```python
from build123d import *

# Parameters (mm, degrees)
SKETCH_1_W          = 10.622879294
SKETCH_1_H          = 7.171059062
EXTRUDE_1_DEPTH     = 6
EXTRUDE_2_DEPTH     = 6
SKETCH_3_W          = 1.75
SKETCH_3_H          = 1.75
CUT_EXTRUDE_1_DEPTH = 4


with BuildPart() as part:
    # 草图1 → 凸台-拉伸1 (new body)
    with BuildSketch(Plane.XY):
        with Locations((2.891532243, 0.829398912)):
            Rectangle(SKETCH_1_W, SKETCH_1_H)
    extrude(amount=EXTRUDE_1_DEPTH)

    # 草图2 → 凸台-拉伸2 (add)
    with BuildSketch(Plane.XY.offset(6)):
        with BuildLine():
            Line((1.830465057, 2.928210333), (3.810000549, 2.928210333))
            ThreePointArc((3.810000549, 2.928210333), (4.51710733, 2.635317114), (4.810000549, 1.928210333))
            Line((4.810000549, 1.928210333), (4.810000549, -0.252824237))
            ThreePointArc((4.810000549, -0.252824237), (4.51710733, -0.959931018), (3.810000549, -1.252824237))
            Line((3.810000549, -1.252824237), (1.830465057, -1.252824237))
            ThreePointArc((1.830465057, -1.252824237), (1.123358276, -0.959931018), (0.830465057, -0.252824237))
            Line((0.830465057, -0.252824237), (0.830465057, 1.928210333))
            ThreePointArc((0.830465057, 1.928210333), (1.123358276, 2.635317114), (1.830465057, 2.928210333))
        make_face()
    extrude(amount=EXTRUDE_2_DEPTH)

    # 草图3 → 切除-拉伸1 (cut)
    with BuildSketch(Plane(origin=(0, 0, 0), x_dir=(-1, 0, 0), z_dir=(0, 0, -1))):
        with Locations((-2.744430707, 0.686146252)):
            Rectangle(SKETCH_3_W, SKETCH_3_H)
    extrude(amount=-CUT_EXTRUDE_1_DEPTH, mode=Mode.SUBTRACT)


solid = part.part
```
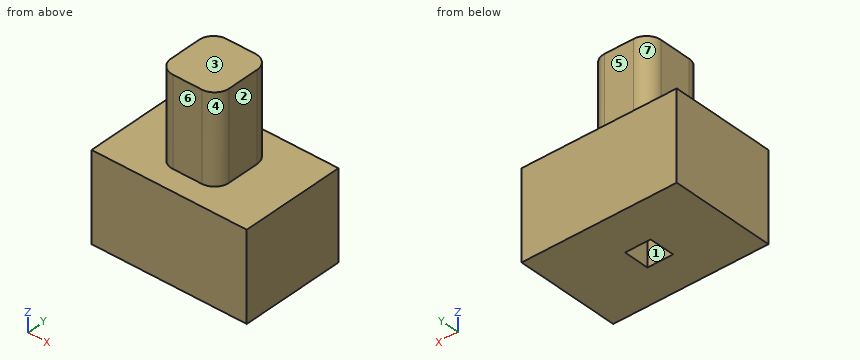
Input: part model. Units: mm. Frame: model coordinates. Face numbers are marked on the shaded views. A direction names the side the tool comes from. Coordinates: 2 decimals unless noted, no trailing zeros. Loops run counter-clockwise (first coordinate to the right, second up) from the corner with the lowest first, then second, coordinate; pieces in that order, holes last. Notation, with made-up numbers: M 3,4.25 L 31,4.25 A26 ccw 31,42.25 Z; hole C 82.5,72 d3. An arc over 180 degrees is marked long. Use a Markdown table: item, result. Add a question column.
1) Line query: L1, parallel to X at y = 0.5, z = 3.5; L2, parallel to Y at x = 3.5, z = 0.5; L3, parallel to X at y = 0.5, z = 9.5. Output: solid intervals per line, ascending. Write a range as from..to.
2) Section A-A, the plane z = 2.5. Return the cut outline in (x, y), plus the area to 3 significant figures.
3) Section C-C, the plane y = 0.25. Return the cut outline in (x, z).
4) Set-up query: the marked faces 4, 5, 6 and 7. Return all of +Z, -Z, +X, -X, +Y, -Y with unobstructed straight access to the full face (end or side cutting, diameter ignored); none if empty.
5) Section D-D, the plane z = 11. Return the cut outline in (x, y), plus the area to 3 significant figures.
6) Draft query along X for the marked faces 1, 2 and 3. Return one class per face: +X half, -X half, draft (parallel to the pull), parting line (faces both ways), or undercut.
7) Pin query (flat end, axial travel): P1, Ø2, axis at x = 3, z = 10, coming from the -Y side; P2, Ø0.9, axis at x = 3, y = 0.5, coming from the -Z side; P3, Ø2.5, axis at y = 1, z = 9, coming from the +X side. Return the tip coordinate at first contact, or that it passes through.
8) Section B-B, the plane x = 3. Return the cut outline in (y, z).
Answer below:
| question | item | result |
|---|---|---|
| 1 | L1 | -2.42..1.87, 3.62..8.2 |
| 1 | L2 | -2.76..-0.19, 1.56..4.41 |
| 1 | L3 | 0.83..4.81 |
| 2 | outline | M -2.42,-2.76 L 8.2,-2.76 L 8.2,4.41 L -2.42,4.41 Z; hole M 1.87,-0.19 L 3.62,-0.19 L 3.62,1.56 L 1.87,1.56 Z |
| 2 | area | 73.1 mm2 |
| 3 | outline | M -2.42,0 L 1.87,0 L 1.87,4 L 3.62,4 L 3.62,0 L 8.2,0 L 8.2,6 L 4.81,6 L 4.81,12 L 0.83,12 L 0.83,6 L -2.42,6 Z |
| 4 | face 4 | +Z, +X, -Y |
| 4 | face 5 | +Z, +X, -X, +Y |
| 4 | face 6 | +Z, +X, -X, -Y |
| 4 | face 7 | +Z, -X, +Y |
| 5 | outline | M 0.83,-0.25 A1 ccw 1.83,-1.25 L 3.81,-1.25 A1 ccw 4.81,-0.25 L 4.81,1.93 A1 ccw 3.81,2.93 L 1.83,2.93 A1 ccw 0.83,1.93 Z |
| 5 | area | 15.8 mm2 |
| 6 | face 1 | undercut |
| 6 | face 2 | +X half |
| 6 | face 3 | draft |
| 7 | P1 | y = -1.25 |
| 7 | P2 | z = 4 |
| 7 | P3 | x = 4.81 |
| 8 | outline | M -2.76,0 L -0.19,0 L -0.19,4 L 1.56,4 L 1.56,0 L 4.41,0 L 4.41,6 L 2.93,6 L 2.93,12 L -1.25,12 L -1.25,6 L -2.76,6 Z |
